CAD build for the part. Positions are in the model's coordinates, mm. A direction names the side the tool comes from. Coordinates: 2 decimals unless noted, no trailing zeros. Order: outer loops, then holes, each group sorted by start corner. A loop starts at its lowest first (then second) coordinate and runs counter-clockwise, first axis right, second up. Notation, with made-up numbers: M -27.5,72 L -22.5,72 A7 ccw -22.5,84 Z; hole C 59,75.5 d5. An arc over 180 degrees is marked long. One line per item, written item: value.
from build123d import *

# Parameters (mm, degrees)
F0_R     = 3.7
F1_DEPTH = 3.9


with BuildPart() as f1:
    # F0 (on Front) → F1 (new body)
    with BuildSketch(Plane.XZ):
        with Locations((0, 0.9)):
            Circle(F0_R)
        Polygon((-0.95, 3.05), (0, 3.05), (0.95, 3.05), (0.95, 1.85), (2.15, 1.85), (2.15, -0.05), (0.95, -0.05), (0.95, -1.25), (-0.95, -1.25), (-0.95, -0.05), (-2.15, -0.05), (-2.15, 1.85), (-0.95, 1.85), align=None, mode=Mode.SUBTRACT)
    extrude(amount=F1_DEPTH)


solid = f1.part
Q1. Pin check, flat tips, straight feed: pin 1 Ø0.6 at (y, z) = (-1.5, 2) entering from +X; pin 2 Ø1.3 at (x, y) = (1.5, -1.5) entering from -Z; pin 3 Ø1.3 at (x, y) = (1.5, -1.5) entering from +Z. Stop position of each tip, or through.
Recorded:
pin 1: stops at x = 3.61
pin 2: stops at z = -2.7
pin 3: stops at z = 4.5
Q2. Which spindle directions (+Z, -Z, +X, -X, +Y, -Y) get a long thin tool onto all of the face, cutting with end or side? Do faces 4 (the face through (2, 0, -1)), 5 (the face through (1.5, -1.9, 1.85)). Say none if no direction does.
Recorded:
face 4: +Z, -Z, +X, -X, +Y
face 5: +Y, -Y
Q3. Slice it at D-D (x = -2.5). List the corners of the cut face in (y, z).
Recorded:
outline: M -3.9,-1.83 L 0,-1.83 L 0,3.63 L -3.9,3.63 Z
Q4. Slice it at C-C (x = 0). List the corners of the cut face in (y, z).
Recorded:
outline: M -3.9,-2.8 L 0,-2.8 L 0,-1.25 L -3.9,-1.25 Z; M -3.9,3.05 L 0,3.05 L 0,4.6 L -3.9,4.6 Z
Q5. Slice it at B-B (y = -2.1). List the corners of the cut face in (x, z).
Recorded:
outline: C 0,0.9 d7.4; hole M -2.15,-0.05 L -0.95,-0.05 L -0.95,-1.25 L 0.95,-1.25 L 0.95,-0.05 L 2.15,-0.05 L 2.15,1.85 L 0.95,1.85 L 0.95,3.05 L -0.95,3.05 L -0.95,1.85 L -2.15,1.85 Z
Q6. Drill centre lines: line 1 along X through (y, z) = (-1.8, 1); line 2 along Z through (x, y) = (0, -2.65); line 3 along Z through (x, y) = (0.75, -2.15). Where is each one in solid material? Low to high.
Recorded:
line 1: x = -3.7 to -2.15, 2.15 to 3.7
line 2: z = -2.8 to -1.25, 3.05 to 4.6
line 3: z = -2.72 to -1.25, 3.05 to 4.52
Q7. Slice it at A-A (z = 0.9). List the corners of the cut face in (x, y), plus the area to 3 significant figures.
Recorded:
outline: M -3.7,-3.9 L -2.15,-3.9 L -2.15,0 L -3.7,0 Z; M 2.15,-3.9 L 3.7,-3.9 L 3.7,0 L 2.15,0 Z
area: 12.1 mm^2
Q8. Mould opens along X. For faces 1 (the face through (0, -2, 3.05)), 2 (the face through (3.53, -1.92, 2.01)), 3 (the face through (2, -3.9, -1)) say: released by +X, released by -X, zero draft, split by the parting line, or undercut.
Recorded:
face 1: undercut
face 2: split by the parting line
face 3: zero draft
